Check sheet for the modelled part. Datum: model origin and axes. Units: mm. Face numbers are marked on the shaded views. Round coordinates to 2 decimals unless told otherwise and drop trailing zeros. Order: outer loops, then holes, each group sorted by start corner. A loop starts at its lowest first (then second) coordinate and runs counter-clockwise, first axis right, second up. Notation, with made-up numbers: (40, 27.25) -> (54, 27.25) arc R14 ccw to (54, 40.25) -> close; hole circle Ø6 at (-24.75, -5). An arc over 180 degrees is marked (long way). Use CSV: the item, a comma, the result in double quotes.
```python
from build123d import *

# Parameters (mm, degrees)
PAD_DEPTH    = 10
SKETCH001_R  = 3.1
POCKET_DEPTH = 17.999765


with BuildPart() as part:
    # Sketch → Pad (new body)
    with BuildSketch(Plane.XY):
        with BuildLine():
            ThreePointArc((-60, -4.472136), (-50, 0), (-60, 4.472136))
            Line((-60, 8.062258), (-60, 4.472136))
            ThreePointArc((-55.850927, 8.998765), (-57.981583, 8.779142), (-60, 8.062258))
            Line((-55.850927, 8.998765), (56.149073, 8.998765))
            ThreePointArc((60, 8.062258), (58.126726, 8.745115), (56.149073, 8.998765))
            Line((60, 8.062258), (60, 4.472136))
            ThreePointArc((60, 4.472136), (50, 0), (60, -4.472136))
            Line((60, -4.472136), (60, -8.062258))
            ThreePointArc((48.516685, -5), (53.681008, -8.696107), (60, -8.062258))
            ThreePointArc((48.516685, -5), (0, 0), (-48.516685, -5))
            ThreePointArc((-60, -8.062258), (-53.681008, -8.696107), (-48.516685, -5))
            Line((-60, -4.472136), (-60, -8.062258))
        make_face()
    extrude(amount=PAD_DEPTH)

    # Sketch001 (on Face4 of Pad) → Pocket (cut, through all)
    with BuildSketch(Plane(origin=(0, 8.998765, 0), x_dir=(-1, 0, 0), z_dir=(0, 1, 0))):
        with Locations((0, 5)):
            Circle(SKETCH001_R)
    extrude(amount=-POCKET_DEPTH, mode=Mode.SUBTRACT)


solid = part.part
```
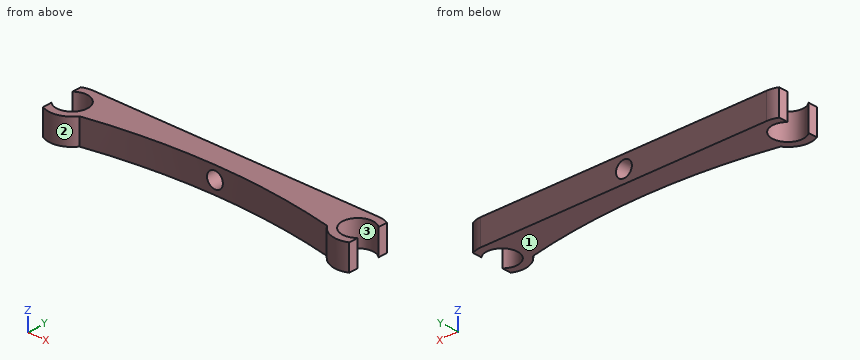
Q1. Sectioned sample at C-C, the plane y = -1.75. Enter the section's corners in (x, z).
Result sheet:
outline,"(-50.26, 0) -> (-28.8, 0) -> (-28.8, 10) -> (-50.26, 10) -> close; (28.8, 0) -> (50.26, 0) -> (50.26, 10) -> (28.8, 10) -> close"
Q2. Sectioned sample at B-B, the plane z = 5. Enter the section's corners in (x, y).
Result sheet:
outline,"(-60, -8.06) arc R9 ccw to (-48.52, -5) arc R237.89 cw to (-3.1, -0.02) -> (-3.1, 9) -> (-55.85, 9) arc R9 ccw to (-60, 8.06) -> (-60, 4.47) arc R6 cw (long way) to (-60, -4.47) -> close; (3.1, -0.02) arc R237.89 cw to (48.52, -5) arc R9 ccw to (60, -8.06) -> (60, -4.47) arc R6 cw (long way) to (60, 4.47) -> (60, 8.06) arc R9 ccw to (56.15, 9) -> (3.1, 9) -> close"
Q3. Mould release check, pull along Y, two halves, no side actions. Record for the marked faces 1, 2 and 3: pulls with the +Y half, pulls with the -Y half, needs draft (parallel to the pull), parting line crosses it, or undercut.
Result sheet:
face 1,"needs draft"
face 2,"pulls with the -Y half"
face 3,"undercut"
Q4. Sectioned sample at D-D, the plane x = -42. Enter the section's corners in (y, z).
Result sheet:
outline,"(-3.74, 0) -> (9, 0) -> (9, 10) -> (-3.74, 10) -> close"
Q5. Go/stop test with flat-tipped pins: pin 1 (3 mm diameter, centred on x = -31.5, z = 8, fed in from -Y); pin 2 (1.5 mm diameter, centred on x = -33.5, z = 8.5, fed in from -Y). Record where each tip stops, or that it passes through.
Result sheet:
pin 1,"stops at y = -2.3"
pin 2,"stops at y = -2.48"
Q6. Scan lines: L1, parallel to Z at x = 0, y = 3.75; L2, parallel to Y at x = -56, z = 4.75; L3, parallel to X at y = 6.25, z = 5.25. Record each from-to range of solid material in increasing order.
Result sheet:
L1,"z = 0 to 1.9, 8.1 to 10"
L2,"y = -9 to -6, 6 to 9"
L3,"x = -60 to -3.09, 3.09 to 60"
Q7. Sectioned sample at A-A, the plane x = -1. Enter the section's corners in (y, z).
Result sheet:
outline,"(0, 0) -> (9, 0) -> (9, 2.07) -> (0, 2.07) -> close; (0, 7.93) -> (9, 7.93) -> (9, 10) -> (0, 10) -> close"
